from build123d import *

# Parameters (mm, degrees)
SKETCH1_W           = 80
SKETCH1_H           = 20
SKETCH1_W_2         = 10
SKETCH1_H_2         = 10
SKETCH1_R           = 2.1
BOSS_EXTRUDE1_DEPTH = 5
SKETCH2_W           = 10
SKETCH2_H           = 3
BOSS_EXTRUDE2_DEPTH = 80
FILLET1_R           = 5
SKETCH3_W           = 2
SKETCH3_H           = 5
CUT_EXTRUDE1_DEPTH  = 53.201532545


with BuildPart() as part:
    # Sketch1 → Boss-Extrude1 (new body)
    # profile 1 of 3: a face of its own
    with BuildSketch(Plane(origin=(0, 0, 0), x_dir=(0, 0, -1), z_dir=(1, 0, 0))):
        Rectangle(SKETCH1_W, SKETCH1_H)
    # profile 2 of 3: a face of its own
    with BuildSketch(Plane(origin=(0, 0, 0), x_dir=(0, 0, -1), z_dir=(1, 0, 0))):
        with Locations((-35, 15)):
            Rectangle(SKETCH1_W_2, SKETCH1_H_2)
        with Locations((-35, 15)):
            Circle(SKETCH1_R, mode=Mode.SUBTRACT)
    # profile 3 of 3: a face of its own
    with BuildSketch(Plane(origin=(0, 0, 0), x_dir=(0, 0, -1), z_dir=(1, 0, 0))):
        with Locations((35, -15)):
            Rectangle(SKETCH1_W_2, SKETCH1_H_2)
        with Locations((35, -15)):
            Circle(SKETCH1_R, mode=Mode.SUBTRACT)
    extrude(amount=BOSS_EXTRUDE1_DEPTH)

    # Sketch2 → Boss-Extrude2 (add)
    with BuildSketch(Plane.XY.offset(40)):
        with Locations((10, 8.5)):
            Rectangle(SKETCH2_W, SKETCH2_H)
        with Locations((10, -8.5)):
            Rectangle(SKETCH2_W, SKETCH2_H)
    extrude(amount=-BOSS_EXTRUDE2_DEPTH)

    # Fillet1
    fillet1_edges = [part.edges().sort_by_distance(p)[0] for p in [
        (2.5, 20, 30),
        (2.5, 20, 40),
        (2.5, -20, -40),
        (2.5, -20, -30),
    ]]
    fillet(fillet1_edges, radius=FILLET1_R - 0.0001)  # a hair under: the kernel refuses the full size

    # Sketch3 → Cut-Extrude1 (cut, through all)
    with BuildSketch(Plane.XZ.offset(10)):
        with Locations((6, 27.5)):
            Rectangle(SKETCH3_W, SKETCH3_H)
        with Locations((6, 9.166666667)):
            Rectangle(SKETCH3_W, SKETCH3_H)
        with Locations((6, -9.166666667)):
            Rectangle(SKETCH3_W, SKETCH3_H)
        with Locations((6, -27.5)):
            Rectangle(SKETCH3_W, SKETCH3_H)
        with Locations((14, 27.5)):
            Rectangle(SKETCH3_W, SKETCH3_H)
        with Locations((14, 9.166666667)):
            Rectangle(SKETCH3_W, SKETCH3_H)
        with Locations((14, -9.166666667)):
            Rectangle(SKETCH3_W, SKETCH3_H)
        with Locations((14, -27.5)):
            Rectangle(SKETCH3_W, SKETCH3_H)
    extrude(amount=-CUT_EXTRUDE1_DEPTH, mode=Mode.SUBTRACT)


solid = part.part
The model under review builds one solid part; all positions refer to its coordinate system, in mm. A direction names the side the tool comes from. Round coordinates to 2 decimals unless told otherwise and drop trailing zeros. Loops run counter-clockwise (first coordinate to the right, second up) from the corner with the lowest first, then second, coordinate; pieces in that order, holes last. Notation, with made-up numbers: (7, 28.25) -> (27, 28.25) arc R10 cw to (27, 35.25) -> close; hole circle Ø1 at (-27, 55). An arc over 180 degrees is marked (long way). Write item = value, one per line. Start each with the question number.
Item 1: To check wall thickness, follow L1, parallel to Z at x = 6.5, y = -8.5; L2, parallel to Y at x = 11.25, z = -9.5; L3, parallel to Y at x = 3.5, z = -35. State the ranges of each line that lie inside material, in increasing order.
Item 2: Insertion check: pin 1 (4 mm diameter, centred on x = 8, z = -10, fed in from +Y); pin 2 (2.5 mm diameter, centred on x = 2.5, y = -12, fed in from +Z); pin 3 (2.5 mm diameter, centred on y = -9, z = -10, fed in from +X). Each pin has a flat end and moves straight along its axis. Give the tip position at first contact, or say it passes through.
Item 3: Take a section at B-B on x = 3.75. Count the separate pieces of the cut face and the enclosed holes in it, plus the area to 3 significant figures.
Item 4: Take a section at D-D on z = 3.5. Give the boundary of the cut face in (x, y), plus the area to 3 significant figures.
Item 5: Mouldability with a two-part tool opening along Z and no side actions: class faces 1 (the flat face through (13, -9, -28)), 2 (the flat face through (6, -9, 6.667)), 3 (the flat face through (4, 3, 40)), 4 (the flat face through (15, 8, -18)) as released by +Z, released by -Z, zero draft, split by the parting line, or undercut.
Item 6: Take a section at C-C on x = 10.75. Give the boundary of the cut face in (y, z).
Item 7: For faces 5 (the flat face through (14, -9, -30)), 6 (the flat face through (7, 8, -28)), 7 (the flat face through (5, -12.7, -34.9)), 8 (the flat face through (5, 12.8, 34)), list the 3-axis set-ups (+Z, -Z, +X, -X, +Y, -Y) from which the entire face can be reached by the end or side of a thin tool; tool diameter is ignored.
Item 8: Take a section at A-A on z = 26.5. Give the boundary of the cut face in (x, y).
Result:
q1.L1 = -40 to -30, -25 to -11.67, -6.67 to 6.67, 11.67 to 25, 30 to 40
q1.L2 = -10 to -7, 7 to 10
q1.L3 = -20 to -17.1, -12.9 to 10
q2.pin_1 = 10
q2.pin_2 = -30
q2.pin_3 = 13
q3.separate_pieces = 1
q3.enclosed_holes = 2
q3.area = 1,750 mm²
q4.outline = (0, -10) -> (15, -10) -> (15, -7) -> (5, -7) -> (5, 7) -> (15, 7) -> (15, 10) -> (0, 10) -> close
q4.area = 160 mm²
q5.face_1 = undercut
q5.face_2 = undercut
q5.face_3 = released by +Z
q5.face_4 = zero draft
q6.outline = (-10, -40) -> (-7, -40) -> (-7, 40) -> (-10, 40) -> close; (7, -40) -> (10, -40) -> (10, 40) -> (7, 40) -> close
q7.face_5 = +X, +Y, -Y
q7.face_6 = +Y, -Y
q7.face_7 = +Z, -Z, +X, -Y
q7.face_8 = +Z, -Z, +X, +Y
q8.outline = (0, -10) -> (5, -10) -> (5, 10) -> (0, 10) -> close; (7, -10) -> (13, -10) -> (13, -7) -> (7, -7) -> close; (7, 7) -> (13, 7) -> (13, 10) -> (7, 10) -> close
